Build history of the part. All positions in model axes, mm. Face numbers are marked on the shaded views. A direction names the side the tool comes from. Round coordinates to 2 decimals unless told otherwise and drop trailing zeros. Loops run counter-clockwise (first coordinate to the right, second up) from the corner with the lowest first, then second, coordinate; pieces in that order, holes last.
from build123d import *

# Parameters (mm, degrees)
SKETCH1_R           = 2
BOSS_EXTRUDE1_DEPTH = 65
SHELL1_T            = -4
SKETCH2_R           = 6
CUT_EXTRUDE1_DEPTH  = 61


with BuildPart() as part:
    # Sketch1 → Boss-Extrude1 (new body)
    with BuildSketch(Plane.XY):
        with BuildLine():
            Line((-33.042, 61), (-33.042, -61))
            ThreePointArc((-33.042, -61), (-31.577533906, -64.535533906), (-28.042, -66))
            Line((-28.042, -66), (33.042, -66))
            Line((33.042, -66), (33.042, 66))
            Line((33.042, 66), (-28.042, 66))
            ThreePointArc((-28.042, 66), (-31.577533906, 64.535533906), (-33.042, 61))
        make_face()
        with Locations((22.958, -55)):
            Circle(SKETCH1_R, mode=Mode.SUBTRACT)
        with Locations((-21.958, 55)):
            Circle(SKETCH1_R, mode=Mode.SUBTRACT)
        with Locations((-21.958, -55)):
            Circle(SKETCH1_R, mode=Mode.SUBTRACT)
        with Locations((22.958, 55)):
            Circle(SKETCH1_R, mode=Mode.SUBTRACT)
    extrude(amount=BOSS_EXTRUDE1_DEPTH)

    # Shell1
    shell1_openings = [part.faces().sort_by_distance(p)[0] for p in [
        (-9.692511302, 0, 0),
    ]]
    offset(amount=SHELL1_T, openings=shell1_openings, kind=Kind.INTERSECTION)

    # Sketch2 → Cut-Extrude1 (cut)
    with BuildSketch(Plane(origin=(0, 0, 0), x_dir=(-1, 0, 0), z_dir=(0, 0, -1))):
        with Locations((-22.958, -55)):
            Circle(SKETCH2_R)
        with Locations((21.958, -55)):
            Circle(SKETCH2_R)
        with Locations((21.958, 55)):
            Circle(SKETCH2_R)
        with Locations((-22.958, 55)):
            Circle(SKETCH2_R)
    extrude(amount=-CUT_EXTRUDE1_DEPTH, mode=Mode.SUBTRACT)


solid = part.part
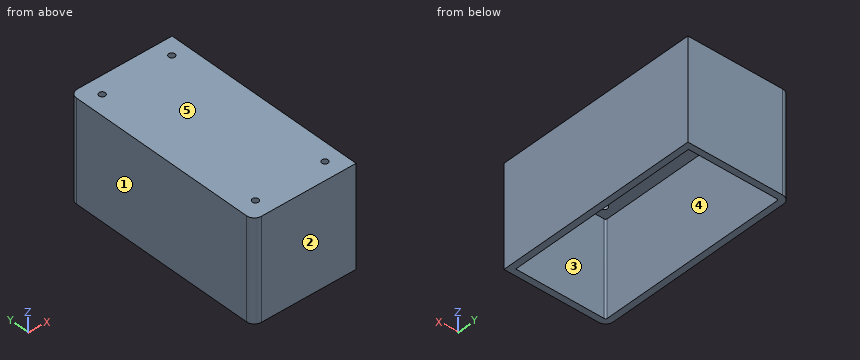
(1) Pin check, flat tip, straight feed: P1, Ø1.5, axis at x = -21.5, y = 23.5, coming from the -Z side. Stop position of the tip, or through.
Responses:
P1: stops at z = 61
(2) Slice it at C-C on x = 11. List the corners of the cut face in (y, z), plus the area to 3 significant figures.
Responses:
outline: (-66, 0) - (-62, 0) - (-62, 61) - (62, 61) - (62, 0) - (66, 0) - (66, 65) - (-66, 65) - close
area: 1,020 mm2
(3) Probe line 1 (X direction, y = -55, z = 62.3); line 2 (Y direction, x = 1.5, z = 17); line 3 (X direction, y = -47.5, z = 41). List the from-to ranges inside material, lowest first.
Responses:
line 1: x = -33.04 to -23.96, -19.96 to 20.96, 24.96 to 33.04
line 2: y = -66 to -62, 62 to 66
line 3: x = -33.04 to -29.04, 29.04 to 33.04
(4) Which spindle directions (+Z, -Z, +X, -X, +Y, -Y) get a long thin tool onto all of the face, cutting with end or side? Do the marked faces 4 and 5. Say none if no direction does.
Responses:
face 4: -Z
face 5: +Z, +X, -X, +Y, -Y
(5) Slice it at A-A on z = 38. List the corners of the cut face in (x, y).
Responses:
outline: (-33.04, -61) arc R5 ccw to (-28.04, -66) - (33.04, -66) - (33.04, 66) - (-28.04, 66) arc R5 ccw to (-33.04, 61) - close; hole (-29.04, -61) arc R1 ccw to (-28.04, -62) - (29.04, -62) - (29.04, 62) - (-28.04, 62) arc R1 ccw to (-29.04, 61) - close
(6) Slice it at B-B on y = -55. List the corners of the cut face in (x, z).
Responses:
outline: (-33.04, 0) - (-29.04, 0) - (-29.04, 61) - (-23.96, 61) - (-23.96, 65) - (-33.04, 65) - close; (-19.96, 61) - (20.96, 61) - (20.96, 65) - (-19.96, 65) - close; (24.96, 61) - (29.04, 61) - (29.04, 0) - (33.04, 0) - (33.04, 65) - (24.96, 65) - close
(7) Pull direction X, two halves, no side cores. Call the marked faces 1, 2 and 3: +X half, -X half, draft (parallel to the pull), parting line (faces both ways), or undercut.
Responses:
face 1: -X half
face 2: draft
face 3: undercut
(8) Slice it at D-D on y = -36. List the corners of the cut face in (x, z).
Responses:
outline: (-33.04, 0) - (-29.04, 0) - (-29.04, 61) - (29.04, 61) - (29.04, 0) - (33.04, 0) - (33.04, 65) - (-33.04, 65) - close
